Verification items for the finished model (mm, model axes). Face numbers are marked on the shaded views. A direction names the side the tool comes from. Give positions to 0.01 mm unless a question says otherwise; leave off trailing zeros. Write each loop counter-clockwise with the first axis right and the second up, starting at its lowest first coordinate (ties: lowest second). Pieces come first, ordered by that corner, then holes. Notation, with made-up numbers: M -40,12.25 L -27,12.25 A23 cw -27,41.25 Z; hole C -18,46 d3. An arc over 180 degrees is marked long. Answer as a JSON object with one key per item and string values.
Autodesk Inventor part; units mm, degrees
ref_plane "YZ Plane" through (0, 0, 0) normal (1, 0, 0) x (0, 1, 0)
ref_plane "XZ Plane" through (0, 0, 0) normal (0, 1, 0) x (-1, 0, 0)
ref_plane "XY Plane" through (0, 0, 0) normal (0, 0, 1) x (1, 0, 0)
sketch "Sketch1" plane through (0, 0, 0) normal (0, 1, 0) x (-1, 0, 0)
  line L0 (25.7234, 17.199) -> (-18.0766, 17.199)
  line L1 (-18.0766, 17.199) -> (-18.0766, -6.201)
  line L2 (-18.0766, -6.201) -> (25.7234, -6.201)
  line L3 (25.7234, -6.201) -> (25.7234, 17.199)
  point P0 (0, 0)
  dimension "d0" = 43.8
  dimension "d1" = 23.4
extrude "Extrusion1" add sketch "Sketch1" along normal blind 1.6
sketch "Sketch2" plane through (0, 1.6, 0) normal (0, 1, 0) x (1, 0, 0)
  line L0 (18.0766, -17.199) -> (18.0766, 6.201)
  line L1 (14.9766, -11.799) -> (14.9766, 1.001)
  line L2 (-25.7234, -17.199) -> (18.0766, -17.199)
  line L3 (14.9766, -11.799) -> (17.4766, -11.799)
  line L4 (17.4766, -11.799) -> (17.4766, 1.001)
  line L5 (17.4766, 1.001) -> (14.9766, 1.001)
  point P0 (0, 0)
  dimension "d6" = 12.8
  dimension "d7" = 0.6
  dimension "d8" = 2.5
  dimension "d9" = 5.4
extrude "Extrusion2" add sketch "Sketch2" along normal blind 2.3
sketch "Sketch3" plane through (0, 3.9, 0) normal (0, 1, 0) x (1, 0, 0)
  line L0 (14.9766, -11.799) -> (17.4766, -11.799)
  line L1 (16.2266, -11.799) -> (16.2266, -9.669)
  circle A0 centre (16.2266, -9.669) radius 0.35
  circle A1 centre (16.2266, -7.539) radius 0.35
  circle A2 centre (16.2266, -5.409) radius 0.35
  circle A3 centre (16.2266, -3.279) radius 0.35
  circle A4 centre (16.2266, -1.149) radius 0.35
  point P0 (0, 0)
  dimension "d12" = 2.13
  dimension "d13" = 0.7
  dimension "d14" = 0.7
  dimension "d15" = 0.7
  dimension "d16" = 0.7
  dimension "d17" = 0.7
  dimension "d19" = 2.13
  dimension "d20" = 2.13
  dimension "d21" = 2.13
  dimension "d22" = 2.13
extrude "Extrusion3" add sketch "Sketch3" along normal blind 6
sketch "Sketch4" plane through (0, 1.6, 0) normal (0, 1, 0) x (1, 0, 0)
  circle A0 centre (-11.7234, -5.499) radius 11
  line L0 (-25.7234, -17.199) -> (18.0766, -17.199)
  line L1 (18.0766, 6.201) -> (-25.7234, 6.201)
  line L2 (-25.7234, 6.201) -> (-25.7234, -17.199)
  point P0 (0, 0)
  dimension "d25" = 22
  dimension "d44" = 14
  dimension "d45" = 11.7
extrude "Extrusion4" add sketch "Sketch4" along normal blind 7.2
sketch "Sketch5" plane through (0, 1.6, 0) normal (0, 1, 0) x (1, 0, 0)
  circle A0 centre (-11.7234, -5.499) radius 11
  line L0 (-1.4006, -1.699) -> (1.0994, -1.699)
  line L1 (1.0994, -1.699) -> (1.0994, -9.299)
  line L2 (1.0994, -9.299) -> (-1.4006, -9.299)
  point P0 (0, 0)
  dimension "d30" = 7.6
  dimension "d31" = 2.5
  dimension "d32" = 2.5
extrude "Extrusion5" add sketch "Sketch5" along normal blind 7.2 contours A0 L0 L1 L2
sketch "Sketch6" plane through (0, 8.8, 0) normal (0, 1, 0) x (1, 0, 0)
  arc A0 (-1.4006, -1.699) -> (-1.4006, -9.299) centre (-11.7234, -5.499) ccw
  circle A1 centre (-11.7234, -5.499) radius 10
  point P0 (0, 0)
  dimension "d35" = 20
extrude "Extrusion6" cut sketch "Sketch6" against normal blind 3.5
sketch "Sketch7" plane through (0, 1.6, 0) normal (0, 1, 0) x (1, 0, 0)
  point P0 (0, 0)
sketch "Sketch8" plane through (0, 1.6, 0) normal (0, 1, 0) x (1, 0, 0)
  line L0 (12.8766, -11.299) -> (12.8766, -1.299)
  line L1 (12.8766, -1.299) -> (2.8766, -1.299)
  line L2 (2.8766, -1.299) -> (2.8766, -11.299)
  line L3 (2.8766, -11.299) -> (12.8766, -11.299)
  line L4 (14.9766, 1.001) -> (14.9766, -11.799)
  line L5 (18.0766, 6.201) -> (-25.7234, 6.201)
  point P0 (0, 0)
  dimension "d38" = 2.1
  dimension "d39" = 10
  dimension "d40" = 10
  dimension "d41" = 7.5
extrude "Extrusion7" add sketch "Sketch8" along normal blind 8.8
sketch "Sketch10" plane through (0, 1.6, 0) normal (0, 1, 0) x (1, 0, 0)
  circle A0 centre (9.0766, -14.199) radius 1.5
  line L0 (18.0766, -17.199) -> (18.0766, 6.201)
  line L1 (-25.7234, -17.199) -> (18.0766, -17.199)
  point P0 (0, 0)
  dimension "d46" = 3
  dimension "d47" = 9
  dimension "d48" = 3
extrude "Extrusion8" add sketch "Sketch10" along normal blind 8
fillet "Fillet1" radius 2 2 edges at (12.8766, 10.4, 6.299) (2.8766, 10.4, 6.299)
sketch "Sketch11" plane through (0, 1.6, 0) normal (0, 1, 0) x (1, 0, 0)
  circle A0 centre (13.4766, -14.699) radius 1.5
  circle A1 centre (13.4766, 3.701) radius 1.5
  circle A2 centre (-22.7234, 3.701) radius 1.5
  circle A3 centre (-22.7234, -14.699) radius 1.5
  line L0 (-25.7234, 6.201) -> (-25.7234, -17.199)
  line L1 (-25.7234, -17.199) -> (18.0766, -17.199)
  point P0 (0, 0)
  dimension "d52" = 3
  dimension "d53" = 3
  dimension "d54" = 21.4
  dimension "d55" = 3
  dimension "d56" = 36.2
  dimension "d57" = 3
  dimension "d58" = 3
  dimension "d59" = 3
  dimension "d60" = 18.4
  dimension "d61" = 2.5
  dimension "d62" = 2.5
  dimension "d64" = 36.2
extrude "Extrusion9" cut sketch "Sketch11" against normal blind 8
sketch "Sketch12" plane through (0, 1.6, 0) normal (0, 1, 0) x (1, 0, 0)
  circle A0 centre (-22.7234, -14.699) radius 1.5
  circle A1 centre (-22.7234, -14.699) radius 1.5
  circle A2 centre (-22.7234, 3.701) radius 1.5
  circle A3 centre (-22.7234, 3.701) radius 1.5
  circle A4 centre (13.4766, 3.701) radius 1.5
  circle A5 centre (13.4766, 3.701) radius 1.5
  circle A6 centre (13.4766, -14.699) radius 1.5
  circle A7 centre (13.4766, -14.699) radius 1.5
  point P0 (0, 0)
properties part number "DS1302"
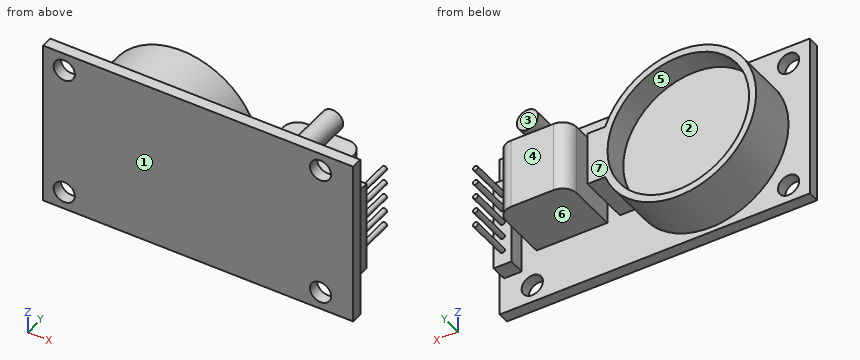
1) Section check B-B on y = 4.5. Record the boundary of the cut face in (x, z).
Completed:
{"outline": "M -1.4,1.7 L 1.1,1.7 L 1.1,9.3 L -1.4,9.3 A11 ccw long Z; M 2.88,1.3 L 12.88,1.3 L 12.88,11.3 L 2.88,11.3 Z; C 9.08,14.2 d3; C 16.23,1.15 d0.7; C 16.23,3.28 d0.7; C 16.23,5.41 d0.7; C 16.23,7.54 d0.7; C 16.23,9.67 d0.7"}
2) Access from +Z, -Z, +X, -X, +Y, -Y to the whole of each face (thin tool, end or side, straight path). Record for the marked faces 3, 4, 5, 6 and 7.
Completed:
{"face 3": "+Z, +X, -X, +Y", "face 4": "+Z, -Z, +X, -X, +Y", "face 5": "+Y", "face 6": "-Z, +Y", "face 7": "+Z, -Z, -X, +Y"}
3) Go/stop test with flat-tipped pins: pin 1 (1.2 mm diameter, centred on y = 2.5, z = 5.5, fed in from -X); pin 2 (12 mm diameter, centred on x = -11.72, z = 5.5, fed in from +Y); pin 3 (6 mm diameter, centred on y = 5, z = 1, fed in from +X). Record where each tip stops, or that it passes through.
Completed:
{"pin 1": "stops at x = -22.72", "pin 2": "stops at y = 5.3", "pin 3": "stops at x = 17.48"}
4) Section check D-D on x = -17. Record the boundary of the cut face in (y, z), and give its area (3 significant figures).
Completed:
{"outline": "M 0,-6.2 L 1.6,-6.2 L 1.6,-4.15 L 8.8,-4.15 L 8.8,-3 L 5.3,-3 L 5.3,13.99 L 8.8,13.99 L 8.8,15.15 L 1.6,15.15 L 1.6,17.2 L 0,17.2 Z", "area": "117 mm2"}
5) Release check for a two-part mould opening along X. For the marked faces 1 and 2 record: pulls with the +X half, pulls with the -X half, needs draft (parallel to the pull), parting line crosses it, or undercut.
Completed:
{"face 1": "needs draft", "face 2": "undercut"}
6) Section check C-C on x = 14.5. Record the boundary of the cut face in (y, z), and give its area (3 significant figures).
Completed:
{"outline": "M 0,-6.2 L 1.6,-6.2 L 1.6,-4.8 L 0,-4.8 Z; M 0,-2.6 L 1.6,-2.6 L 1.6,13.6 L 0,13.6 Z; M 0,15.8 L 1.6,15.8 L 1.6,17.2 L 0,17.2 Z", "area": "30.4 mm2"}
7) Thickness scan on L1, parallel to X at y = 6.75, z = 3.75; L2, parallel to X at y = 3, z = 9; L3, parallel to Y at x = -13.5, z = 14. Record the ranges inside material, lowest first.
Completed:
{"L1": "x = -22.58 to -21.57, -1.88 to 1.1, 2.88 to 12.88", "L2": "x = -22.15 to 1.1, 2.88 to 12.88, 14.98 to 17.48", "L3": "y = 0 to 5.3"}
8) Section check A-A on y = 6.5. Count the separate pieces of the cut face and the enclosed holes in it, and give its area (3 significant figures).
Completed:
{"separate pieces": "8", "enclosed holes": "1", "area": "191 mm2"}
